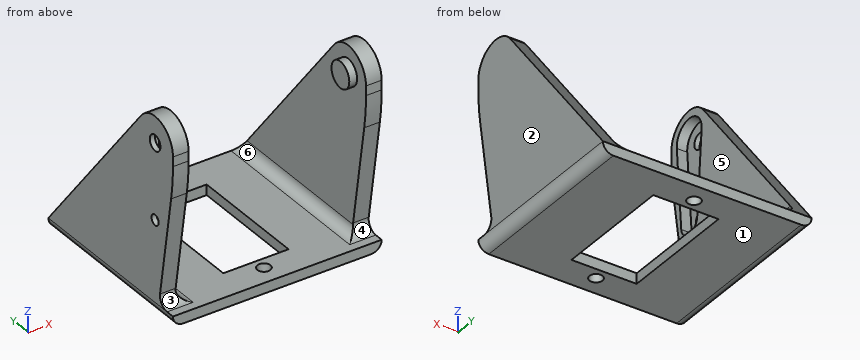
```python
from build123d import *

# Parameters (mm, degrees)
SKETCH_1_W          = 40
SKETCH_1_H          = 35
SKETCH_1_R          = 1.25
SKETCH_1_W_2        = 12.5
SKETCH_1_H_2        = 23
EXTRUDE_1_DEPTH     = 2
EXTRUDE_2_DEPTH     = 3
CUT_EXTRUDE_1_DEPTH = 2
SKETCH_4_R          = 2.5
EXTRUDE_3_DEPTH     = 1.5
CUT_EXTRUDE_2_DEPTH = 58.22979993
FILLET_1_R          = 40
SKETCH_6_R          = 1.5
CUT_EXTRUDE_3_DEPTH = 10
SKETCH_7_R          = 1
CUT_EXTRUDE_4_DEPTH = 10
FILLET_2_R          = 2


with BuildPart() as part:
    # 草图1 → 凸台-拉伸1 (new body)
    with BuildSketch(Plane.XY):
        Rectangle(SKETCH_1_W, SKETCH_1_H)
        with Locations((0, 13.75)):
            Circle(SKETCH_1_R, mode=Mode.SUBTRACT)
        with Locations((0, -13.75)):
            Circle(SKETCH_1_R, mode=Mode.SUBTRACT)
        Rectangle(SKETCH_1_W_2, SKETCH_1_H_2, mode=Mode.SUBTRACT)
    extrude(amount=EXTRUDE_1_DEPTH)

    # 草图2 → 凸台-拉伸2 (add)
    with BuildSketch(Plane.ZY.offset(20)):
        with BuildLine():
            Line((2, -17.5), (32, -17.5))
            ThreePointArc((32, -17.5), (36.724288943, -14.13740465), (35.094229072, -8.572437595))
            Line((35.094229072, -8.572437595), (2, 17.5))
            Line((2, 17.5), (2, -17.5))
        make_face()
    extrude_2 = extrude(amount=-EXTRUDE_2_DEPTH)

    # 草图3 → 切除-拉伸1 (cut)
    with BuildSketch(Plane(origin=(-17, 0, 0), x_dir=(0, 0, -1), z_dir=(1, 0, 0))):
        with BuildLine():
            Line((-15.82421875, -10.256876965), (-31.7265625, -9.0106975))
            ThreePointArc((-31.7265625, -9.0106975), (-35.5, -12.5), (-31.7265625, -15.9893025))
            Line((-31.7265625, -15.9893025), (-15.82421875, -14.743123035))
            ThreePointArc((-15.82421875, -14.743123035), (-13.75, -12.5), (-15.82421875, -10.256876965))
        make_face()
    extrude(amount=-CUT_EXTRUDE_1_DEPTH, mode=Mode.SUBTRACT)

    # 镜向3: 凸台-拉伸2 across plane
    add(extrude_2.mirror(Plane(origin=(0, 0, 0), x_dir=(0, 0, 1), z_dir=(1, 0, 0))))

    # 草图4 → 凸台-拉伸3 (add)
    with BuildSketch(Plane.ZY.offset(-17)):
        with Locations((32, -12.5)):
            Circle(SKETCH_4_R)
    extrude(amount=EXTRUDE_3_DEPTH)

    # 草图5 → 切除-拉伸2 (cut, through all)
    with BuildSketch(Plane(origin=(20, 0, 0), x_dir=(0, 0, -1), z_dir=(1, 0, 0))):
        Polygon((-2, -17.5), (-2, -13.5), (-27, -17.5), align=None)
    extrude(amount=-CUT_EXTRUDE_2_DEPTH, mode=Mode.SUBTRACT)

    # 圆角1
    fillet_1_edges = [part.edges().sort_by_distance(p)[0] for p in [
        (-18.5, -17.5, 27),
        (18.5, -17.5, 27),
    ]]
    fillet(fillet_1_edges, radius=FILLET_1_R)

    # 草图6 → 切除-拉伸3 (cut)
    with BuildSketch(Plane(origin=(-19, 0, 0), x_dir=(0, 0, -1), z_dir=(1, 0, 0))):
        with Locations((-32, -12.5)):
            Circle(SKETCH_6_R)
    extrude(amount=-CUT_EXTRUDE_3_DEPTH, mode=Mode.SUBTRACT)

    # 草图7 → 切除-拉伸4 (cut)
    with BuildSketch(Plane(origin=(-19, 0, 0), x_dir=(0, 0, -1), z_dir=(1, 0, 0))):
        with Locations((-17.5, -12.5)):
            Circle(SKETCH_7_R)
    extrude(amount=-CUT_EXTRUDE_4_DEPTH, mode=Mode.SUBTRACT)

    # 圆角2
    fillet_2_edges = [part.edges().sort_by_distance(p)[0] for p in [
        (17, 2, 2),
        (-17, 2, 2),
        (20, 0, 0),
        (-20, 0, 0),
        (18.5, -13.5, 2),
        (-18.5, -13.5, 2),
    ]]
    fillet(fillet_2_edges, radius=FILLET_2_R - 0.0001)  # a hair under: the kernel refuses the full size


solid = part.part
```
Build history of the part. All positions in model axes, mm. Face numbers are marked on the shaded views. A direction names the side the tool comes from. Give positions to 0.01 mm unless a question says otherwise; leave off trailing zeros. Order: outer loops, then holes, each group sorted by start corner. A loop starts at its lowest first (then second) coordinate and runs counter-clockwise, first axis right, second up. Notation, with made-up numbers: M 0.25,22 L 33.25,22 A30 ccw 33.25,53 Z; hole C 19,86.5 d1. An arc over 180 degrees is marked long. Write item = value, one per line. Start each with the question number.
(1) Two-plate mould, pull along Z, no slides. Class the marked faces 1, 2 and 3: released by +Z, released by -Z, zero draft, split by the parting line, or undercut.
(2) Probe L1, parallel to X at y = -11, z = 29.5; L2, parallel to X at y = -5.5, z = 11; L3, parallel to Z at x = 14.5, y = 2. List the from-to ranges inside material, lowest first. Write a range as [from, to].
(3) Slice it at A-A on x = 0. Write the cut outline in (y, z), plus the area to 3 significant figures.
(4) Pin check, flat tips, straight feed: pin 1 Ø2 at (x, y) = (0, -13.75) entering from -Z; pin 2 Ø1.6 at (y, z) = (-3.5, 0.5) entering from -X; pin 3 Ø2 at (x, y) = (12, -8) entering from +Z; pin 4 Ø10 at (x, z) = (12.5, 8.5) entering from +Y. Stop position of each tip, or through.
(5) Slice it at D-D on z = 17.5. Write the cut outline in (x, y).
(6) Slice it at C-C on z = 12. Write the cut outline in (x, y).
(7) Slice it at B-B on y = 13.75. Write the cut outline in (x, z).
(8) Which spindle directions (+Z, -Z, +X, -X, +Y, -Y) get a long thin tool onto all of the face, cutting with end or side? Do the marked faces 4, 5 and 6. Say none if no direction does.
Responses:
q1.face_1 = released by -Z
q1.face_2 = zero draft
q1.face_3 = undercut
q2.L1 = [-20, -19], [17, 20]
q2.L2 = [-20, -17], [17, 20]
q2.L3 = [0, 2]
q3.outline = M -17.5,0 L -15,0 L -15,2 L -17.5,2 Z; M -12.5,0 L -11.5,0 L -11.5,2 L -12.5,2 Z; M 11.5,0 L 12.5,0 L 12.5,2 L 11.5,2 Z; M 15,0 L 17.5,0 L 17.5,2 L 15,2 Z
q3.area = 14.0 mm2
q4.pin_1 = through
q4.pin_2 = -19.87
q4.pin_3 = 2
q4.pin_4 = 14.1
q5.outline = M -20,-15.98 L -17,-15.98 L -17,-14.87 L -19,-14.87 L -19,-13.5 L -20,-13.5 Z; M -20,-11.5 L -19,-11.5 L -19,-10.13 L -17,-10.13 L -17,5.29 L -20,5.29 Z; M 17,-15.98 L 20,-15.98 L 20,5.29 L 17,5.29 Z
q6.outline = M -20,-15.1 L -17,-15.1 L -17,9.62 L -20,9.62 Z; M 17,-15.1 L 20,-15.1 L 20,9.62 L 17,9.62 Z
q7.outline = M -20,2 A2 ccw -18,0 L -1.25,0 L -1.25,2 L -15,2 A2 cw -17,4 L -17,6.76 L -20,6.76 Z; M 1.25,0 L 18,0 A2 ccw 20,2 L 20,6.76 L 17,6.76 L 17,4 A2 cw 15,2 L 1.25,2 Z
q8.face_4 = +X, -X, -Y
q8.face_5 = +Z, +Y, -Y
q8.face_6 = +Y, -Y
